```python
from build123d import *

# Parameters (mm, degrees)
F1_DEPTH       = 16
F2_DEPTH       = 18
F4_D           = 21
F4_CBORE_D     = 30
F4_CBORE_DEPTH = 6
F6_DEPTH       = 30
F8_D           = 13


with BuildPart() as f1:
    # F0 (on Front) → F1 (new body)
    with BuildSketch(Plane.XZ):
        with BuildLine():
            Line((-48.5, 13.5), (48.5, 13.5))
            Line((48.5, 13.5), (48.5, 58.997409))
            ThreePointArc((48.5, 58.997409), (0, 70.5), (-48.5, 58.997409))
            Line((-48.5, 58.997409), (-48.5, 13.5))
        make_face()
        with BuildLine():
            ThreePointArc((-28.378378, 41.561164), (0, 46.5), (28.378378, 41.561164))
            ThreePointArc((28.378378, 41.561164), (34.412043, 28.770742), (21.621622, 22.737077))
            ThreePointArc((21.621622, 22.737077), (0, 26.5), (-21.621622, 22.737077))
            ThreePointArc((-21.621622, 22.737077), (-34.412043, 28.770742), (-28.378378, 41.561164))
        make_face(mode=Mode.SUBTRACT)
    extrude(amount=F1_DEPTH)

    # F0 (on Front) → F2 (join)
    with BuildSketch(Plane.XZ):
        with BuildLine():
            ThreePointArc((-48.5, -58.997409), (0, -70.5), (48.5, -58.997409))
            Line((48.5, -58.997409), (48.5, 13.5))
            Line((48.5, 13.5), (-48.5, 13.5))
            Line((-48.5, 13.5), (-48.5, -58.997409))
        make_face()
    extrude(amount=F2_DEPTH)

    # F4 (through all)
    with Locations(Plane.XZ.offset(18)):
        with Locations((0, -39.5)):
            CounterBoreHole(F4_D / 2, F4_CBORE_D / 2, F4_CBORE_DEPTH)

    # F5 (on face) → F6 (join)
    with BuildSketch(Plane.XZ.offset(18)):
        with BuildLine():
            Line((-48.5, 13.5), (-48.5, -58.997409))
            ThreePointArc((-48.5, -58.997409), (-40.630053, -62.565972), (-32.5, -65.493932))
            Line((-32.5, -65.493932), (-32.5, 13.5))
            Line((-32.5, 13.5), (-48.5, 13.5))
        make_face()
        with BuildLine():
            ThreePointArc((32.5, -65.493932), (40.630053, -62.565972), (48.5, -58.997409))
            Line((48.5, -58.997409), (48.5, 13.5))
            Line((48.5, 13.5), (32.5, 13.5))
            Line((32.5, 13.5), (32.5, -65.493932))
        make_face()
    extrude(amount=F6_DEPTH)

    # F8 (through all)
    with Locations(Plane(origin=(-48.5, 0, 0), x_dir=(0, -1, 0), z_dir=(-1, 0, 0))):
        with Locations((33, 0.5)):
            Hole(F8_D / 2)


solid = f1.part
```
For this review, take the finished solid that the model builds, in its own axes (mm). A direction names the side the tool comes from. Coordinates: 2 decimals unless noted, no trailing zeros. Order: outer loops, then holes, each group sorted by start corner. A loop starts at its lowest first (then second) coordinate and runs counter-clockwise, first axis right, second up. Notation, with made-up numbers: (11.5, -25) - (38.5, -25) arc R3 ccw to (38.5, -20) - close; hole circle Ø5 at (59.5, -14). An arc over 180 degrees is marked (long way). Answer as a JSON object with one key per item and string values. Group by question number.
1. For probe 1 along Z at (x, y) = (0, -14); probe 2 along Z at (x, y) = (0, -4.75); probe 3 along X at (y, z) = (-39, 4), list the stretches that pass through material, from the lowest coordinate up.
2. The part is to be moulded in two halves that separate along X. For faces 5 (the cylindrical face through (-40.74, -32.79, -62.52)), 6 (the flat face through (40, -48, -25)), 7 (the flat face through (32.5, -33, -25)), say which applies: pulls with the +X half, pulls with the -X half, needs draft (parallel to the pull), parting line crosses it, or undercut.
3. We need section A-A on x = 0. State the section outline as (y, z) points.
4. Clearance check with flat-ended pins moving along their axes: P1, Ø24, axis at x = 4, z = -34, coming from the -Y side; P2, Ø21, axis at y = -33, z = 0.5, coming from the -X side; P3, Ø12.5, axis at x = 0, z = -39.5, coming from the -Y side; P4, Ø10, axis at x = -24, y = -21.5, coming from the -Z side. State where each tip first meets the part, or that it passes through.
5. We need section D-D on x = 30. State the section outline as (y, z) points, then the cut area to 3 significant figures.
6. We need section C-C on y = -33. State the section outline as (x, z) points.
7. We need section B-B on z = -39.5. State the section outline as (x, y) points.
8. For faces 1 (the flat face through (-10.2, -12, -42.6)), 2 (the cylindrical face through (0.3, -7.9, 26.5)), 3 (the flat face through (-32.5, -33, -27)), 4 (the flat face through (11.5, -17.6, 13.5)), list the 3-axis set-ups (+Z, -Z, +X, -X, +Y, -Y) from which the entire face can be reached by the end or side of a thin tool; tool diameter is ignored.
Final values:
{
 "1": {"probe 1": "-70.5 to -54.5, -24.5 to 26.5, 46.5 to 70.5", "probe 2": "-70.5 to -50, -29 to 26.5, 46.5 to 70.5", "probe 3": "-48.5 to -32.5, 32.5 to 48.5"},
 "2": {"face 5": "pulls with the -X half", "face 6": "needs draft", "face 7": "undercut"},
 "3": {"outline": "(-18, -70.5) - (0, -70.5) - (0, -50) - (-12, -50) - (-12, -54.5) - (-18, -54.5) - close; (-18, -24.5) - (-12, -24.5) - (-12, -29) - (0, -29) - (0, 26.5) - (-16, 26.5) - (-16, 13.5) - (-18, 13.5) - close; (-16, 46.5) - (0, 46.5) - (0, 70.5) - (-16, 70.5) - close"},
 "4": {"P1": "y = -18", "P2": "x = -48.5", "P3": "through", "P4": "z = -68.55"},
 "5": {"outline": "(-18, -66.25) - (0, -66.25) - (0, 23.49) - (-16, 23.49) - (-16, 13.5) - (-18, 13.5) - close; (-16, 40.81) - (0, 40.81) - (0, 66.25) - (-16, 66.25) - close", "area": "2,000 mm²"},
 "6": {"outline": "(-48.5, -59) arc R108 ccw to (-32.5, -65.49) - (-32.5, -6) - (-48.5, -6) - close; (-48.5, 7) - (-32.5, 7) - (-32.5, 13.5) - (-48.5, 13.5) - close; (32.5, -65.49) arc R108 ccw to (48.5, -59) - (48.5, -6) - (32.5, -6) - close; (32.5, 7) - (48.5, 7) - (48.5, 13.5) - (32.5, 13.5) - close"},
 "7": {"outline": "(-48.5, -48) - (-32.5, -48) - (-32.5, -18) - (-15, -18) - (-15, -12) - (-10.5, -12) - (-10.5, 0) - (-48.5, 0) - close; (10.5, -12) - (15, -12) - (15, -18) - (32.5, -18) - (32.5, -48) - (48.5, -48) - (48.5, 0) - (10.5, 0) - close"},
 "8": {"face 1": "-Y", "face 2": "+Y, -Y", "face 3": "+Z, -Z, -Y", "face 4": "+Z, +X, -X, -Y"}
}
